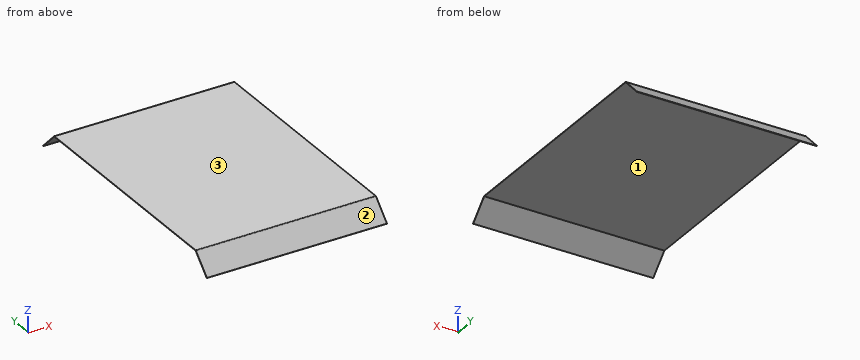
Autodesk Inventor part; units mm, degrees
ref_plane "YZ Plane" through (0, 0, 0) normal (1, 0, 0) x (0, 1, 0)
ref_plane "XZ Plane" through (0, 0, 0) normal (0, 1, 0) x (-1, 0, 0)
ref_plane "XY Plane" through (0, 0, 0) normal (0, 0, 1) x (1, 0, 0)
sketch "Sketch1" plane through (0, 0, 0) normal (0, 0, 1) x (1, 0, 0)
  line L0 (-739.5, -950) -> (739.5, -950)
  line L1 (739.5, -950) -> (739.5, 950)
  line L2 (739.5, 950) -> (-739.5, 950)
  line L3 (-739.5, 950) -> (-739.5, -950)
  line L4 (-739.5, -950) -> (739.5, 950) construction
  line L5 (739.5, -950) -> (-739.5, 950) construction
  point P0 (0, 0)
  dimension "d0" = 1479
  dimension "d1" = 1900
extrude "Plate1" add sketch "Sketch1" along normal blind 3
sketch "Sketch2" plane through (739.5, 947.8787, 0.8787) normal (0, 0.7071068, 0.7071068) x (-1, 0, 0)
  line L0 (1479, 0) -> (0, 0)
  line L1 (0, 0) -> (0, -212)
  line L2 (0, -212) -> (1479, -212)
  line L3 (1479, -212) -> (1479, 0)
edge flange "Flange1" height 212 angle 45 thickness 3 bend radius 5 thickness toward (0, 0.7071068, 0.7071068) relief round relief width 3 relief depth 1.5 corner gap 5 corner form 0 edges at (0, 950, 0) (0, -950, 0) wall of the first edge with corners at (-739.5, 947.8787, 0.8787) (739.5, 947.8787, 0.8787) (739.5, 1097.7853, -149.028) (-739.5, 1097.7853, -149.028)
bend "Bend1"
corner "Corner1"
sketch "Sketch4" plane through (739.5, 1097.7853, -149.028) normal (0, -0.7071068, -0.7071068) x (-1, 0, 0)
  line L0 (25, -40) -> (25, -25) construction
  line L1 (25, -25) -> (225, -25) construction
  line L2 (225, -25) -> (225, -40) construction
  line L3 (225, -40) -> (25, -40) construction
  line L4 (1479, 0) -> (0, 0)
  line L5 (0, -208.6863) -> (0, 0)
  point P0 (739.5, -881.6301)
  dimension "d13" = 200
  dimension "d14" = 15
  dimension "d15" = 25
  dimension "d16" = 25
mark "Mark1"
equation "\"d2\" = Thickness"
equation "\"d3\" = BendReliefWidth"
equation "\"d4\" = BendReliefDepth"
equation "\"d5\" = MinimumRemnant"
equation "\"d6\" = TransitionRadius"
equation "\"d9\" = BendRadius"
equation "\"d10\" = CornerReliefSize"
equation "\"d11\" = GapSize"
equation "\"d12\" = JacobiRadiusSize"
equation "\"BendReliefWidth\" = Thickness"
equation "\"BendReliefDepth\" = 0.5 * Thickness"
equation "\"CornerReliefSize\" = 4 * Thickness"
equation "\"MinimumRemnant\" = 2 * Thickness"
equation "\"TransitionRadius\" = BendRadius"
equation "\"JacobiRadiusSize\" = BendRadius"
equation "\"GapSize\" = Thickness"
properties part number "BSH 011 floor" material "09g2s"
Geometry: final body of the model. Coordinates: model frame, mm. Face numbers are marked on the shaded views. Round coordinates to 2 decimals unless told otherwise and drop trailing zeros. Loops run counter-clockwise (first coordinate to the right, second up) from the corner with the lowest first, then second, coordinate; pieces in that order, holes last. Notation, with made-up numbers: M 42,15.25 L 72,15.25 A21 ccw 72,21.25 Z; hole C 14.5,8 d8. An arc over 180 degrees is marked long. Put each result on its own line as item: value. Start each with the question number.
(1) Contact query for flat-ended pins moving along their axis: pin 1 Ø10 at (x, y) = (532, 405.5) entering from -Z; pin 2 Ø1.5 at (x, z) = (-203.5, -102) entering from +Y; pin 3 Ø10 at (x, z) = (518, -110.5) entering from -Y. Output: stop coordinate, or through.
(2) Section query C-C (y = -60). Return loops of the section in (x, z).
(3) Section query A-A (x = -225.5). Return loops of the section in (y, z).
(4) Material intervals for line 1 along Z through (x, y) = (275, -633); line 2 along Y through (x, z) = (414, -48); line 3 along Y through (x, z) = (-375, -93.5), sorted ascending. Write a range as [from, to].
(5) Section query B-B (z = -60). Return loops of the section in (x, y).
(6) Draft query along Y for the marked faces 1, 2 and 3. Return one class per face: +Y half, -Y half, draft (parallel to the pull), parting line (faces both ways), or undercut.
Findings below:
1. pin 1: stops at z = 0
1. pin 2: stops at y = 1055.75
1. pin 3: stops at y = -1068.5
2. outline: M -739.5,0 L 739.5,0 L 739.5,3 L -739.5,3 Z
3. outline: M -1099.91,-146.91 L -1097.79,-149.03 L -950.22,-1.46 A5 cw -946.69,0 L 946.69,0 A5 cw 950.22,-1.46 L 1097.79,-149.03 L 1099.91,-146.91 L 952.34,0.66 A8 ccw 946.69,3 L -946.69,3 A8 ccw -952.34,0.66 Z
4. line 1: z = [0, 3]
4. line 2: y = [-1001, -996.76], [996.76, 1001]
4. line 3: y = [-1046.5, -1042.26], [1042.26, 1046.5]
5. outline: M -739.5,-1013 L 739.5,-1013 L 739.5,-1008.76 L -739.5,-1008.76 Z; M -739.5,1008.76 L 739.5,1008.76 L 739.5,1013 L -739.5,1013 Z
6. face 1: undercut
6. face 2: -Y half
6. face 3: draft
